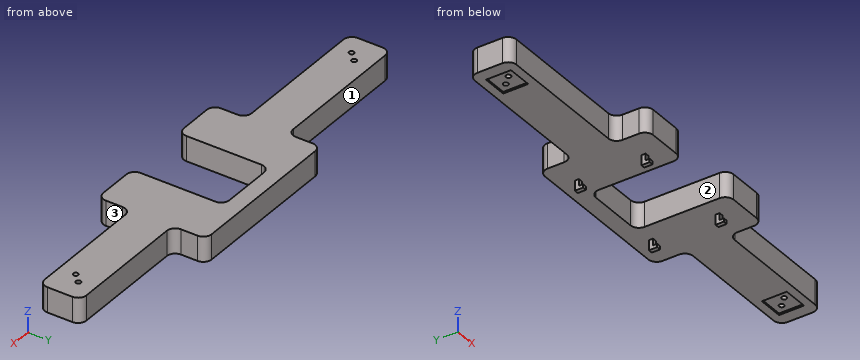
```python
from build123d import *

# Parameters (mm, degrees)
F1_DEPTH  = 150
F2_R      = 50
F3_W      = 150
F3_H      = 150
F4_DEPTH  = 10
F6_R      = 15
F7_DEPTH  = 200
F8_R      = 15
F9_DEPTH  = 200
F10_W     = 25
F10_H     = 50
F11_DEPTH = 60
F12_W     = 25
F12_H     = 40
F13_DEPTH = 100
F14_W     = 25
F14_H     = 40
F15_DEPTH = 100
F16_W     = 25
F16_H     = 40
F17_DEPTH = 1000


# Not quite as in the source:
# - two fillets or chamfers of one size are made in one step
# - a feature names something its author has since deleted; it is built from what else it names


with BuildPart() as f1:
    # F0 (on Top) → F1 (new body)
    with BuildSketch(Plane.XY):
        Polygon((0, 250), (0, 0), (900, 0), (900, -200), (1200, -200), (1200, 350), (1600, 350), (1600, -200), (1900, -200), (1900, 0), (2700, 0), (2700, 250), (1900, 250), (1900, 450), (900, 450), (900, 250), align=None)
    extrude(amount=F1_DEPTH)

    # F2
    f2_edges = [f1.edges().sort_by_distance(p)[0] for p in [
        (1600, 350, 75),
        (1600, -200, 75),
        (1900, -200, 75),
        (1900, 450, 75),
        (900, 450, 75),
        (900, 250, 75),
        (0, 250, 75),
        (0, 0, 75),
        (900, 0, 75),
        (900, -200, 75),
        (1200, -200, 75),
        (1200, 350, 75),
        (1900, 0, 75),
        (2700, 0, 75),
        (2700, 250, 75),
        (1900, 250, 75),
    ]]
    fillet(f2_edges, radius=F2_R)

    # F3 (on face) → F4 (cut)
    with BuildSketch(Plane(origin=(0, 0, 0), x_dir=(1, 0, 0), z_dir=(0, 0, -1))):
        with Locations((150, -125)):
            Rectangle(F3_W, F3_H)
        with Locations((2550, -125)):
            Rectangle(F3_W, F3_H)
    extrude(amount=-F4_DEPTH, mode=Mode.SUBTRACT)

    # F6 (on face) → F7 (cut)
    with BuildSketch(Plane(origin=(0, 0, 10), x_dir=(1, 0, 0), z_dir=(0, 0, -1))):
        with Locations((175, -150)):
            Circle(F6_R)
        with Locations((125, -100)):
            Circle(F6_R)
    extrude(amount=-F7_DEPTH, mode=Mode.SUBTRACT)

    # F8 (on face) → F9 (cut)
    with BuildSketch(Plane(origin=(0, 0, 10), x_dir=(1, 0, 0), z_dir=(0, 0, -1))):
        with Locations((2525, -100)):
            Circle(F8_R)
        with Locations((2575, -150)):
            Circle(F8_R)
    extrude(amount=-F9_DEPTH, mode=Mode.SUBTRACT)

    # F10 (on face) → F11 (join)
    with BuildSketch(Plane(origin=(0, 0, 0), x_dir=(1, 0, 0), z_dir=(0, 0, -1))):
        with Locations((1077.5, 75)):
            Rectangle(F10_W, F10_H)
        with Locations((1722.5, 75)):
            Rectangle(F10_W, F10_H)
        with Locations((1077.5, -325)):
            Rectangle(F10_W, F10_H)
        with Locations((1722.5, -325)):
            Rectangle(F10_W, F10_H)
    extrude(amount=F11_DEPTH)

    # F12 (on face) → F13 (cut)
    with BuildSketch(Plane(origin=(1065, 0, 0), x_dir=(0, -1, 0), z_dir=(-1, 0, 0))):
        with Locations((87.5, -20)):
            Rectangle(F12_W, F12_H)
    extrude(amount=-F13_DEPTH, mode=Mode.SUBTRACT)

    # F14 (on face) → F15 (cut)
    with BuildSketch(Plane(origin=(1710, 0, 0), x_dir=(0, -1, 0), z_dir=(-1, 0, 0))):
        with Locations((87.5, -20)):
            Rectangle(F14_W, F14_H)
    extrude(amount=-F15_DEPTH, mode=Mode.SUBTRACT)

    # F16 (on face) → F17 (cut)
    with BuildSketch(Plane(origin=(1065, 0, 0), x_dir=(0, -1, 0), z_dir=(-1, 0, 0))):
        with Locations((-312.5, -20)):
            Rectangle(F16_W, F16_H)
    extrude(amount=-F17_DEPTH, mode=Mode.SUBTRACT)


solid = f1.part
```
Design review of the part built by this model. Coordinates are the model's own, in mm. Face numbers are marked on the shaded views. A direction names the side the tool comes from. Coordinates: 2 decimals unless noted, no trailing zeros. Write each loop counter-clockwise with the first axis right and the second up, starting at its lowest first coordinate (ties: lowest second). Pieces come first, ordered by that corner, then holes.
1) Add section B-B (z = 73). State how many separate pieces and enclosed holes the cut face has, plus the area to 3 significant figures.
2) Insertion check: pin 1 (5 mm diameter, centred on x = 141.5, z = 4.5, fed in from -Y); pin 2 (6 mm diameter, centred on x = 2336, z = 118.5, fed in from +Y); pin 3 (7.5 mm diameter, centred on x = 1071.5, z = -20, fed in from +Y). Each pin has a flat end and moves straight along its axis. Give the tip position at first contact, or say it passes through.
3) To check wall thickness, follow L1, parallel to X at y = 100, z = 59; L2, parallel to X at y = 150, z = 92; L3, parallel to Y at x = 2575, z = 90.5. State the ranges of each line that lie inside material, in increasing order.
4) Add section C-C (x = 750). Write out the cut boundary in (y, z).
5) Machinability: for the marked faces 1, 2 and 3, which of the approach directions +Z, -Z, +X, -X, +Y, -Y give a long, thin tool a straight path to every point of the face, cutting with its end or side? Answer none if there is none.
6) Add section A-A (x = 1039.5). Write out the cut boundary in (y, z).
Check result:
1. separate pieces: 1
1. enclosed holes: 4
1. area: 850,000 mm2
2. pin 1: stops at y = 0
2. pin 2: stops at y = 250
2. pin 3: stops at y = 350
3. L1: x = 0 to 110, 140 to 1200, 1600 to 2510, 2540 to 2700
3. L2: x = 0 to 160, 190 to 1200, 1600 to 2560, 2590 to 2700
3. L3: y = 0 to 135, 165 to 250
4. outline: (0, 0) - (250, 0) - (250, 150) - (0, 150) - close
5. face 1: +Z, -Z, -X, +Y
5. face 2: +Z, -Z, -Y
5. face 3: +Z, -Z, +X, -Y
6. outline: (-200, 0) - (450, 0) - (450, 150) - (-200, 150) - close
